For this review, take the finished solid that the model builds, in its own axes (mm). Face numbers are marked on the shaded views. A direction names the side the tool comes from. Coordinates: 2 decimals unless noted, no trailing zeros. Loops run counter-clockwise (first coordinate to the right, second up) from the corner with the lowest first, then second, coordinate; pieces in that order, holes last. Notation, with made-up numbers: M 63,22 L 75,22 A10 cw 75,30 Z; hole C 83,83 d9. An arc over 180 degrees is marked long. Write each question's results on one line, items separated by ' | '. Start each with the question number.
```python
from build123d import *

# Parameters (mm, degrees)
SKETCH1_W           = 142.24
SKETCH1_H           = 91.44
BOSS_EXTRUDE1_DEPTH = 40.64
SKETCH3_W           = 101.6
SKETCH3_H           = 76.2
BOSS_EXTRUDE2_DEPTH = 38.1
SKETCH4_W           = 70.885711102
SKETCH4_H           = 34.639527003
CUT_EXTRUDE2_DEPTH  = 97.79
SKETCH5_W           = 90.875163882
SKETCH5_H           = 2.870686322
CUT_EXTRUDE3_DEPTH  = 97.79
SKETCH8_W           = 91.28479526
SKETCH8_H           = 30.48
BOSS_EXTRUDE4_DEPTH = 28.575
SKETCH9_W           = 37.704579212
SKETCH9_H           = 3.084273822
CUT_EXTRUDE4_DEPTH  = 28.321
SKETCH10_W          = 3.65161605
SKETCH10_H          = 25.540665071
CUT_EXTRUDE5_DEPTH  = 14.097
SKETCH2_W           = 87.63
SKETCH2_H           = 36.83
CUT_EXTRUDE6_DEPTH  = 225.933
SKETCH12_W          = 91.44
SKETCH12_H          = 40.64
BOSS_EXTRUDE5_DEPTH = 2.667
SKETCH13_W          = 6.720820965
SKETCH13_H          = 6.891818051
SKETCH13_R          = 1.25
SKETCH13_W_2        = 8.363974295
BOSS_EXTRUDE6_DEPTH = 43.815
SKETCH14_R          = 1.25
CUT_EXTRUDE7_DEPTH  = 13.843


with BuildPart() as part:
    # Sketch1 → Boss-Extrude1 (new body)
    with BuildSketch(Plane(origin=(0, 0, 0), x_dir=(1, 0, 0), z_dir=(0, 1, 0))):
        Rectangle(SKETCH1_W, SKETCH1_H)
    extrude(amount=BOSS_EXTRUDE1_DEPTH)

    # Sketch3 → Boss-Extrude2 (add)
    with BuildSketch(Plane(origin=(0, 40.64, 0), x_dir=(1, 0, 0), z_dir=(0, 1, 0))):
        with Locations((-20.32, 0.743974295)):
            Rectangle(SKETCH3_W, SKETCH3_H)
    extrude(amount=BOSS_EXTRUDE2_DEPTH)

    # Sketch4 → Cut-Extrude2 (cut)
    with BuildSketch(Plane.ZY.offset(71.12)):
        with Locations((-0.546263413, 58.617752018)):
            Rectangle(SKETCH4_W, SKETCH4_H)
    extrude(amount=-CUT_EXTRUDE2_DEPTH, mode=Mode.SUBTRACT)

    # Sketch5 → Cut-Extrude3 (cut)
    with BuildSketch(Plane.XY.offset(37.356025705)):
        with Locations((-20.498494518, 61.797236891)):
            Rectangle(SKETCH5_W, SKETCH5_H)
    extrude(amount=-CUT_EXTRUDE3_DEPTH, mode=Mode.SUBTRACT)

    # Sketch8 → Boss-Extrude4 (add)
    with BuildSketch(Plane(origin=(30.48, 0, 0), x_dir=(0, 0, -1), z_dir=(1, 0, 0))):
        with Locations((-0.07760237, 55.88)):
            Rectangle(SKETCH8_W, SKETCH8_H)
    extrude(amount=BOSS_EXTRUDE4_DEPTH)

    # Sketch9 → Cut-Extrude4 (cut)
    with BuildSketch(Plane(origin=(59.055, 0, 0), x_dir=(0, 0, -1), z_dir=(1, 0, 0))):
        with Locations((0.04199785, 65.042136911)):
            Rectangle(SKETCH9_W, SKETCH9_H)
        with Locations((0.04199785, 61.957863089)):
            Rectangle(SKETCH9_W, SKETCH9_H)
        Polygon((-18.810291756, 63.5), (-44.40800215, 63.5), (-44.40800215, 40.64), (44.49199785, 40.64), (44.49199785, 63.5), (18.894287456, 63.5), (18.894287456, 60.415726178), (-18.810291756, 60.415726178), align=None)
    extrude(amount=-CUT_EXTRUDE4_DEPTH, mode=Mode.SUBTRACT)

    # Sketch10 → Cut-Extrude5 (cut)
    with BuildSketch(Plane(origin=(0, 71.12, 0), x_dir=(1, 0, 0), z_dir=(0, 1, 0))):
        with Locations((32.305808025, -0.58046966)):
            Rectangle(SKETCH10_W, SKETCH10_H)
    extrude(amount=-CUT_EXTRUDE5_DEPTH, mode=Mode.SUBTRACT)

    # Sketch2 → Cut-Extrude6 (cut)
    with BuildSketch(Plane(origin=(71.12, 0, 0), x_dir=(0, 0, -1), z_dir=(1, 0, 0))):
        with Locations((0, 20.32)):
            Rectangle(SKETCH2_W, SKETCH2_H)
    extrude(amount=-CUT_EXTRUDE6_DEPTH, mode=Mode.SUBTRACT)

    # Sketch12 → Boss-Extrude5 (add)
    with BuildSketch(Plane(origin=(71.12, 0, 0), x_dir=(0, 0, -1), z_dir=(1, 0, 0))):
        with Locations((0, 20.32)):
            Rectangle(SKETCH12_W, SKETCH12_H)
    extrude(amount=-BOSS_EXTRUDE5_DEPTH)

    # Sketch13 → Boss-Extrude6 (add)
    # profile 1 of 2: a face of its own
    with BuildSketch(Plane.ZY.offset(71.12)):
        with Locations((-42.204384778, 44.085909026)):
            Rectangle(SKETCH13_W, SKETCH13_H)
        with Locations((-41.837350795, 43.997172438)):
            Circle(SKETCH13_R, mode=Mode.SUBTRACT)
    # profile 2 of 2: a face of its own
    with BuildSketch(Plane.ZY.offset(71.12)):
        with Locations((41.538012853, 44.085909026)):
            Rectangle(SKETCH13_W_2, SKETCH13_H)
        with Locations((41.130421673, 43.997172438)):
            Circle(SKETCH13_R, mode=Mode.SUBTRACT)
    extrude(amount=-BOSS_EXTRUDE6_DEPTH)

    # Sketch14 → Cut-Extrude7 (cut)
    with BuildSketch(Plane(origin=(59.055, 0, 0), x_dir=(0, 0, -1), z_dir=(1, 0, 0))):
        with Locations((-41.323220525, 67.518632332)):
            Circle(SKETCH14_R)
        with Locations((40.552025118, 67.518632332)):
            Circle(SKETCH14_R)
    extrude(amount=-CUT_EXTRUDE7_DEPTH, mode=Mode.SUBTRACT)


solid = part.part
```
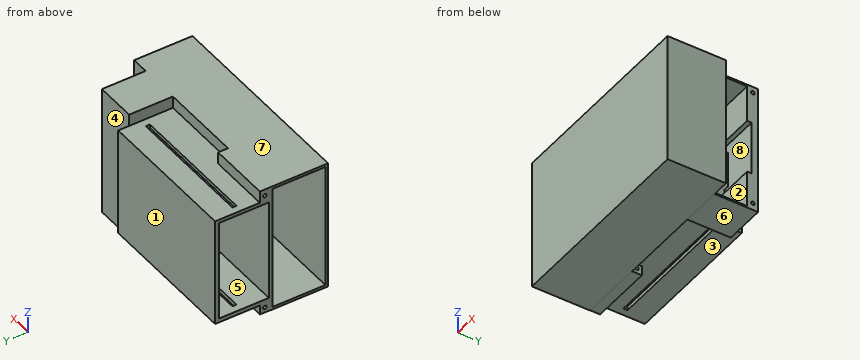
Q1. Insertion check: P1, Ø24, axis at y = 65.5, z = -2.5, coming from the +X side (3 decimals); P2, Ø1.8, axis at x = 32.5, y = 62, coming from the -Z side; P3, Ø3.5, axis at x = -56.5, z = -43.5, coming from the +Y side. Each pin has a flat end and moves straight along its axis. Give the tip position at first contact, or say it passes through.
Q2. Take a section at B-B, the plane z = -3. Give the boundary of the cut face in (x, y) (3 decimals), then the cut area to 3 significant figures.
Q3. Take a section at D-D, the plane x = -34. Give the boundary of the cut face in (y, z) (3 decimals), then the cut area to 3 significant figures.
Q4. For the marked faces 4, 5, 6, 7 and 8, list the 3-axis set-ups (+Z, -Z, +X, -X, +Y, -Y) from which the entire face can be reached by the end or side of a thin tool; tool diameter is ignored.
Q5. To check wall thickness, follow line 1 along Y through (x, z) = (52.5, 20) (3 decimals); line 2 along Y through (x, z) = (49.5, -5) (3 decimals); line 3 along Z through (x, y) = (-6.5, 55.5). State the ranges of each line that lie inside material, in increasing order.
Q6. Take a section at A-A, the plane x = 4. Give the boundary of the cut face in (y, z) (3 decimals), then the cut area to 3 significant figures.
Q7. The part is to be moulded in two halves that separate along Y. For the marked faces 1, 2 and 3, say which applies: pulls with the +Y half, pulls with the -Y half, needs draft (parallel to the pull), parting line crosses it, or undercut.
Q8. Take a section at C-C, the plane y = 51. Give the boundary of the cut face in (x, z) (3 decimals).
Results:
1) P1: x = 59.055 | P2: z = -45.56 | P3: y = 47.53
2) outline: M -71.12,0 L 71.12,0 L 71.12,40.64 L 30.734,40.64 L 30.734,57.023 L 30.48,57.023 L 30.48,78.74 L -71.12,78.74 L -71.12,75.938 L 26.67,75.938 L 26.67,41.298 L -71.12,41.298 L -71.12,38.735 L 68.453,38.735 L 68.453,1.905 L -71.12,1.905 Z; M 34.132,66.584 L 59.055,66.584 L 59.055,71.12 L 34.132,71.12 Z | area: 1,240 mm^2
3) outline: M 0,-45.72 L 40.64,-45.72 L 40.64,-45.565 L 47.532,-45.565 L 47.532,-38.844 L 60.362,-38.844 L 60.362,-35.989 L 41.298,-35.989 L 41.298,34.897 L 60.362,34.897 L 60.362,37.356 L 47.532,37.356 L 47.532,45.72 L 0,45.72 Z; M 63.233,-38.844 L 78.74,-38.844 L 78.74,37.356 L 63.233,37.356 L 63.233,34.897 L 75.938,34.897 L 75.938,-35.989 L 63.233,-35.989 Z; hole M 1.905,-43.815 L 38.735,-43.815 L 38.735,43.815 L 1.905,43.815 Z; hole C 43.997,-41.837 d2.5; hole C 43.997,41.13 d2.5 | area: 1,020 mm^2
4) face 4: +Z, -Z, +X, +Y | face 5: -X | face 6: -Z, +X, -X, +Y | face 7: +Z, +X, -X, +Y, -Y | face 8: +X
5) line 1: 0 to 1.905, 38.735 to 40.64, 63.5 to 71.12 | line 2: 0 to 1.905, 38.735 to 40.64, 66.584 to 71.12 | line 3: -38.84 to -35.99, 34.9 to 37.36
6) outline: M 0,-45.72 L 40.64,-45.72 L 40.64,-38.844 L 60.362,-38.844 L 60.362,-35.989 L 41.298,-35.989 L 41.298,34.897 L 60.362,34.897 L 60.362,37.356 L 40.64,37.356 L 40.64,45.72 L 0,45.72 Z; M 63.233,-38.844 L 78.74,-38.844 L 78.74,37.356 L 63.233,37.356 L 63.233,34.897 L 75.938,34.897 L 75.938,-35.989 L 63.233,-35.989 Z; hole M 1.905,-43.815 L 38.735,-43.815 L 38.735,43.815 L 1.905,43.815 Z | area: 921 mm^2
7) face 1: pulls with the +Y half | face 2: undercut | face 3: needs draft
8) outline: M -71.12,-38.844 L 30.48,-38.844 L 30.48,-45.565 L 59.055,-45.565 L 59.055,-44.492 L 30.734,-44.492 L 30.734,44.408 L 59.055,44.408 L 59.055,45.72 L 30.48,45.72 L 30.48,37.356 L -71.12,37.356 L -71.12,34.897 L 26.67,34.897 L 26.67,-35.989 L -71.12,-35.989 Z
